```python
from build123d import *

# Parameters (mm, degrees)
SKETCH1_R                    = 14
BOSS_EXTRUDE1_DEPTH          = 3
FILLET1_R                    = 3
M3_CLEARANCE_HOLE1_D         = 3.2
CSK_FOR_M3_SFHCS1_AT_2_COUNT = 2
CSK_FOR_M3_SFHCS1_AT_2_PITCH = 32.126856443
BOSS_EXTRUDE3_START          = -3
BOSS_EXTRUDE3_DEPTH          = 3
M3_CLEARANCE_HOLE2_D         = 3.2
BOSS_EXTRUDE4_DEPTH          = 3
FILLET2_R                    = 1


with BuildPart() as part:
    # Sketch1 → Boss-Extrude1 (new body)
    with BuildSketch(Plane.XY):
        with BuildLine():
            Line((-7.713858659, 20.231714727), (-27.069818728, -0.727922061))
            Line((-27.069818728, -0.727922061), (-40.727922061, -0.727922061))
            Line((-40.727922061, -0.727922061), (-44.727922061, -0.727922061))
            ThreePointArc((-44.727922061, -0.727922061), (-48.263455967, -2.192388155), (-49.727922061, -5.727922061))
            Line((-49.727922061, -5.727922061), (-49.727922061, -19.727922061))
            ThreePointArc((-49.727922061, -19.727922061), (-48.263455967, -23.263455967), (-44.727922061, -24.727922061))
            Line((-44.727922061, -24.727922061), (-40.727922061, -24.727922061))
            Line((-40.727922061, -24.727922061), (-24.76951664, -24.727922061))
            ThreePointArc((-24.76951664, -24.727922061), (-24.748737342, -24.748737342), (-24.727922061, -24.76951664))
            Line((-24.727922061, -24.76951664), (-24.727922061, -40.727922061))
            Line((-24.727922061, -40.727922061), (-24.727922061, -44.727922061))
            ThreePointArc((-24.727922061, -44.727922061), (-23.263455967, -48.263455967), (-19.727922061, -49.727922061))
            Line((-19.727922061, -49.727922061), (-5.727922061, -49.727922061))
            ThreePointArc((-5.727922061, -49.727922061), (-2.192388155, -48.263455967), (-0.727922061, -44.727922061))
            Line((-0.727922061, -44.727922061), (-0.727922061, -40.727922061))
            Line((-0.727922061, -40.727922061), (-0.727922061, -27.069818728))
            Line((-0.727922061, -27.069818728), (20.231714727, -7.713858659))
            ThreePointArc((20.231714727, -7.713858659), (21.420744979, -5.069187867), (20.337771086, -2.379346963))
            Line((20.337771086, -2.379346963), (-2.379346963, 20.337771086))
            ThreePointArc((-2.379346963, 20.337771086), (-5.069187867, 21.420744979), (-7.713858659, 20.231714727))
        make_face()
        with Locations((-12.727922061, -12.727922061)):
            Circle(SKETCH1_R, mode=Mode.SUBTRACT)
        with BuildLine():
            Line((-44.727922061, -22.727922061), (-40.727922061, -22.727922061))
            ThreePointArc((-40.727922061, -22.727922061), (-38.606601718, -21.849242405), (-37.727922061, -19.727922061))
            Line((-37.727922061, -19.727922061), (-37.727922061, -5.727922061))
            ThreePointArc((-37.727922061, -5.727922061), (-38.606601718, -3.606601718), (-40.727922061, -2.727922061))
            Line((-40.727922061, -2.727922061), (-44.727922061, -2.727922061))
            ThreePointArc((-44.727922061, -2.727922061), (-46.849242405, -3.606601718), (-47.727922061, -5.727922061))
            Line((-47.727922061, -5.727922061), (-47.727922061, -19.727922061))
            ThreePointArc((-47.727922061, -19.727922061), (-46.849242405, -21.849242405), (-44.727922061, -22.727922061))
        make_face(mode=Mode.SUBTRACT)
        with BuildLine():
            Line((-19.727922061, -37.727922061), (-5.727922061, -37.727922061))
            ThreePointArc((-5.727922061, -37.727922061), (-3.606601718, -38.606601718), (-2.727922061, -40.727922061))
            Line((-2.727922061, -40.727922061), (-2.727922061, -44.727922061))
            ThreePointArc((-2.727922061, -44.727922061), (-3.606601718, -46.849242405), (-5.727922061, -47.727922061))
            Line((-5.727922061, -47.727922061), (-19.727922061, -47.727922061))
            ThreePointArc((-19.727922061, -47.727922061), (-21.849242405, -46.849242405), (-22.727922061, -44.727922061))
            Line((-22.727922061, -44.727922061), (-22.727922061, -40.727922061))
            ThreePointArc((-22.727922061, -40.727922061), (-21.849242405, -38.606601718), (-19.727922061, -37.727922061))
        make_face(mode=Mode.SUBTRACT)
    extrude(amount=BOSS_EXTRUDE1_DEPTH)

    # Fillet1
    # the kernel refuses this fillet: 3 mm, written as the material it adds along each edge
    with BuildSketch(Plane(origin=(-0.727922061, -27.069818728, 0), x_dir=(0.734653136445674, 0.6784429004054313, 0), z_dir=(0, 0, 1)), Plane(origin=(-27.069818728, -0.727922061, 0), x_dir=(-1, 0, 0), z_dir=(0, 0, 1))) as fillet1_piece_1:
        with BuildLine():
            CenterArc((FILLET1_R * 0.437699212924, -FILLET1_R), FILLET1_R, 90, 47.277914711)
            Line((-FILLET1_R * 0.296953923521, -FILLET1_R * 0.321557099595), (-FILLET1_R * 0.31164698625, -FILLET1_R * 0.307988241586))
            Line((-FILLET1_R * 0.31164698625, -FILLET1_R * 0.307988241586), (-FILLET1_R * 0.00875398425848, FILLET1_R * 0.02))
            Line((-FILLET1_R * 0.00875398425848, FILLET1_R * 0.02), (FILLET1_R * 0.437699212924, FILLET1_R * 0.02))
            Line((FILLET1_R * 0.437699212924, FILLET1_R * 0.02), (FILLET1_R * 0.437699212924, 0))
        make_face()
    extrude(amount=3)
    with BuildSketch(Plane(origin=(-24.727922061, -24.76951664, 0), x_dir=(-0.7071067811869401, 0.707106781186155, 0), z_dir=(0, 0, 1))) as fillet1_piece_2:
        with BuildLine():
            CenterArc((1.798711298, 2.443929389), FILLET1_R, 225, 9.552090636)
            Line((-0.322609046, 0.322609046), (-0.365035452, 0.280182639))
            Line((-0.365035452, 0.280182639), (-0.042426407, -0.042426407))
            Line((-0.042426407, -0.042426407), (0.000103806, -0.05999991))
            ThreePointArc((0.000103806, -0.05999991), (0.029411809, -0.059974557), (0.024025864, -0.048878588))
            Line((0.024025864, -0.048878588), (0.058823617, 0))
        make_face()
    extrude(amount=3)

    # M3 Clearance Hole1 (through all)
    with Locations(Plane(origin=(0, 0, 0), x_dir=(-1, 0, 0), z_dir=(0, 0, -1))):
        with Locations((0, 0)):
            Hole(M3_CLEARANCE_HOLE1_D / 2)

    # Sketch5 → CSK for M3 SFHCS1 (revolve, cut)
    with BuildSketch(Plane(origin=(-4.995642054, 17.721475995, 0), x_dir=(0, 1, 0), z_dir=(1, 0, 0))):
        Polygon((0, 0), (0, 3), (1.6, 3), (1.6, 1.76), (3.36, 0), align=None)
    csk_for_m3_sfhcs1 = revolve(axis=Axis((-4.995642054, 17.721475995, -6.35), (0, 0, 1)), mode=Mode.SUBTRACT)

    # CSK for M3 SFHCS1 at 2: CSK for M3 SFHCS1 ×2
    with Locations(*[Vector(0.7071067811865475, -0.7071067811865477, 0) * (i * CSK_FOR_M3_SFHCS1_AT_2_PITCH) for i in range(1, CSK_FOR_M3_SFHCS1_AT_2_COUNT)]):
        add(csk_for_m3_sfhcs1, mode=Mode.SUBTRACT)

    # Sketch8 → Boss-Extrude3 (add)
    with BuildSketch(Plane.XY.offset(3).offset(BOSS_EXTRUDE3_START)):
        with BuildLine():
            Line((-49.727922061, 2.272077939), (-49.727922061, -5.727922061))
            ThreePointArc((-49.727922061, -5.727922061), (-48.263455967, -2.192388155), (-44.727922061, -0.727922061))
            Line((-44.727922061, -0.727922061), (-37.983715361, -0.727922061))
            Line((-37.983715361, -0.727922061), (-41.431833634, 4.688627679))
            ThreePointArc((-41.431833634, 4.688627679), (-46.486413634, 6.592517611), (-49.727922061, 2.272077939))
        make_face()
        with BuildLine():
            Line((-41.431833634, -30.144471802), (-37.983715361, -24.727922061))
            Line((-37.983715361, -24.727922061), (-44.727922061, -24.727922061))
            ThreePointArc((-44.727922061, -24.727922061), (-48.263455967, -23.263455967), (-49.727922061, -19.727922061))
            Line((-49.727922061, -19.727922061), (-49.727922061, -27.727922061))
            ThreePointArc((-49.727922061, -27.727922061), (-46.486413634, -32.048361734), (-41.431833634, -30.144471802))
        make_face()
    boss_extrude3 = extrude(amount=BOSS_EXTRUDE3_DEPTH)

    # Sketch10 → CSK for M3 SFHCS2 (revolve, cut)
    with BuildSketch(Plane(origin=(-45.227922061, 2.272077939, 0), x_dir=(0, 1, 0), z_dir=(1, 0, 0))):
        Polygon((0, 0), (0, 3), (1.6, 3), (1.6, 1.76), (3.36, 0), align=None)
    csk_for_m3_sfhcs2 = revolve(axis=Axis((-45.227922061, 2.272077939, -6.35), (0, 0, 1)), mode=Mode.SUBTRACT)

    # M3 Clearance Hole2 (through all)
    with Locations(Plane(origin=(0, 0, 0), x_dir=(-1, 0, 0), z_dir=(0, 0, -1))):
        with Locations((45.227922061, -27.727922061)):
            m3_clearance_hole2 = Hole(M3_CLEARANCE_HOLE2_D / 2)

    # Mirror1: Boss-Extrude3, CSK for M3 SFHCS2, M3 Clearance Hole2 across plane
    add(boss_extrude3.mirror(Plane(origin=(0, 0, 0), x_dir=(0, 0, 1), z_dir=(-0.7071067811865475, 0.7071067811865477, 0))))
    add(csk_for_m3_sfhcs2.mirror(Plane(origin=(0, 0, 0), x_dir=(0, 0, 1), z_dir=(-0.7071067811865475, 0.7071067811865477, 0))), mode=Mode.SUBTRACT)
    add(m3_clearance_hole2.mirror(Plane(origin=(0, 0, 0), x_dir=(0, 0, 1), z_dir=(-0.7071067811865475, 0.7071067811865477, 0))), mode=Mode.SUBTRACT)

    # Sketch13 → Boss-Extrude4 (add)
    with BuildSketch(Plane(origin=(0, 0, 0), x_dir=(-1, 0, 0), z_dir=(0, 0, -1))):
        with BuildLine():
            Line((-21.199587058, -6.257681448), (-6.502213015, -46.762834838))
            ThreePointArc((-6.502213015, -46.762834838), (-6.726271236, -44.587483093), (-5.898401366, -42.563381125))
            Line((-5.898401366, -42.563381125), (-17.692883881, -10.058436905))
            Line((-17.692883881, -10.058436905), (-20.231714727, -7.713858659))
            ThreePointArc((-20.231714727, -7.713858659), (-20.802903641, -7.043764039), (-21.199587058, -6.257681448))
        make_face()
        with BuildLine():
            Line((10.058436905, 17.692883881), (7.713858659, 20.231714727))
            ThreePointArc((7.713858659, 20.231714727), (7.043764039, 20.802903641), (6.257681448, 21.199587058))
            Line((6.257681448, 21.199587058), (46.762834838, 6.502213015))
            ThreePointArc((46.762834838, 6.502213015), (44.587483093, 6.726271236), (42.563381125, 5.898401366))
            Line((42.563381125, 5.898401366), (10.058436905, 17.692883881))
        make_face()
        with BuildLine():
            Line((30.909902577, -48.409902577), (48.409902577, -30.909902577))
            ThreePointArc((48.409902577, -30.909902577), (46.534165101, -32.034165101), (44.349937703, -32.141440325))
            Line((44.349937703, -32.141440325), (32.141440325, -44.349937703))
            ThreePointArc((32.141440325, -44.349937703), (32.034165101, -46.534165101), (30.909902577, -48.409902577))
        make_face()
    extrude(amount=-BOSS_EXTRUDE4_DEPTH)

    # Fillet2
    fillet2_edges = [part.edges().sort_by_distance(p)[0] for p in [
        (-37.983715361, -0.727922061, 1.5),
        (-37.983715361, -24.727922061, 1.5),
        (-0.727922061, -37.983715361, 1.5),
        (-24.727922061, -37.983715361, 1.5),
        (17.692883881, -10.058436905, 1.5),
        (5.898401366, -42.563381125, 1.5),
        (-42.563381125, 5.898401366, 1.5),
        (-10.058436905, 17.692883881, 1.5),
        (-32.141440325, -44.349937703, 1.5),
        (-44.349937703, -32.141440325, 1.5),
    ]]
    fillet(fillet2_edges, radius=FILLET2_R)


solid = part.part
```
Build history of the part. All positions in model axes, mm. A direction names the side the tool comes from. Give positions to 0.01 mm unless a question says otherwise; leave off trailing zeros. Loops run counter-clockwise (first coordinate to the right, second up) from the corner with the lowest first, then second, coordinate; pieces in that order, holes last. Notation, with made-up numbers: (31, 79.5) -> (61, 79.5) arc R29 ccw to (61, 109.5) -> close; hole circle Ø2 at (78, 4). An arc over 180 degrees is marked (long way). One line per question, with ' | ' between items.
Q1. Cut at B-B, the plane z = 1. Count the separate pieces of the cut face and the enclosed holes in it, plus the area to 3 significant figures.
Filled sheet:
separate pieces: 1 | enclosed holes: 13 | area: 2,030 mm²
Q2. Pull direction Y, two halves, no side cores. Call faces 3 (the cylindrical face through (4.89, -48.89, 1.48)), 4 (the cylindrical face through (-12.74, 15.89, 1.52)), 5 (the flat face through (-49.728, -13, 1)): pulls with the +Y half, pulls with the -Y half, needs draft (parallel to the pull), parting line crosses it, or undercut.
Filled sheet:
face 3: pulls with the -Y half | face 4: undercut | face 5: needs draft
Q3. Cut at A-A, the plane y = -11. Write the cut outline in (x, z).
Filled sheet:
outline: (-49.73, 0) -> (-47.73, 0) -> (-47.73, 3) -> (-49.73, 3) -> close; (-37.73, 0) -> (-26.62, 0) -> (-26.62, 3) -> (-37.73, 3) -> close; (1.17, 0) -> (19.48, 0) -> (19.48, 3) -> (1.17, 3) -> close
Q4. Drop flat-ended pins along their axis: pin 1 (0.9 mm diameter, centred on x = -33, z = 1, fed in from +Y); pin 2 (0.9 mm diameter, centred on x = -14.5, z = 1, fed in from +Y); pin 3 (0.9 mm diameter, centred on y = -28.5, z = 1.5, fed in from -X). Give the stop position or say it passes through.
Filled sheet:
pin 1: stops at y = 11.66 | pin 2: stops at y = 18.37 | pin 3: stops at x = -49.72
Q5. Tool access for faces 1 (the flat face through (-17, -27, 0)), 2 (the flat face through (-0.728, -33, 1)): list every direction of +Z, -Z, +X, -X, +Y, -Y with a clear straight run to the whole face (end or side of a thin tool).
Filled sheet:
face 1: -Z, +X, -X, +Y, -Y | face 2: +Z, -Z
Q6. Drill centre lines: line 1 along X through (y, z) = (-25, 0.7); line 2 along X through (y, z) = (-18.5, 1.55); line 3 along X through (y, z) = (-33, 0.9). Where is each one in solid material? Low to high. Write a range as [from, to].
Filled sheet:
line 1: x = [-49.73, -38.12], [-24.74, -19.47], [-5.99, 1.51], [12.27, 14.4] | line 2: x = [-49.73, -47.73], [-37.73, -25.48], [0.03, 8.55], [14.63, 16.76] | line 3: x = [-46.32, -43.43], [-24.73, -0.73], [9.37, 11.5]
